from build123d import *

# Parameters (mm, degrees)
F0_R     = 33.4136580184
F1_DEPTH = 38.0875840783
F3_R     = 0.3813665803


with BuildPart() as f1:
    # F0 (on Top) → F1 (new body)
    with BuildSketch(Plane.XY):
        Circle(F0_R)
    extrude(amount=F1_DEPTH)

    # F2: F1 across plane


with BuildPart() as f1_1:
    add(f1.part)
    add(f1.part.mirror(Plane.XY))

    # F3
    f3_edges = [f1_1.edges().sort_by_distance(p)[0] for p in [
        (-33.413658, 0, -38.087584),
        (-33.413658, 0, 38.087584),
    ]]
    fillet(f3_edges, radius=F3_R)


solid = f1_1.part
Can you work these out from the model? Positions are in its coordinate system, mm. Give positions to 0.01 mm unless a question says otherwise; leave off trailing zeros. Loops run counter-clockwise (first coordinate to the right, second up) from the corner with the lowest first, then second, coordinate; pieces in that order, holes last. Notation, with made-up numbers: (-40, 67.25) -> (-35, 67.25) arc R8 cw to (-35, 79.25) -> close; hole circle Ø3 at (32, 49.25). An arc over 180 degrees is marked (long way). Write item = value, one per line.
1) Will these pins go through, and if not, where does the flat tip stop? pin 1 (10 mm diameter, centred on x = -13.5, z = -20.5, fed in from +Y); pin 2 (8 mm diameter, centred on y = 17, z = -23, fed in from +X); pin 3 (12 mm diameter, centred on y = 12.5, z = -22.5, fed in from +X).
Check result:
pin_1 = 32.31
pin_2 = 30.78
pin_3 = 32.78
2) I need wall thicknesses on L1, parallel to Y at x = -5, z = -14.5; L2, parallel to Y at x = 2, z = 3. Which ranges of each line are inside material? Lowest first, please. Write a range as from..to.
Check result:
L1 = -33.04..33.04
L2 = -33.35..33.35
3) Suppose I cut it at A-A on z = -13. Write out the boundary of the cut face in (x, y).
Check result:
outline = circle Ø66.83 at (0, 0)
4) Thinking about a two-plate mould opening in Y: for faces 1 (the flat face through (0, 0, -38.088)), 2 (the cylindrical face through (-26.516, -20.332, 0.528)), which applies, released by +Y, released by -Y, zero draft, split by the parting line, or undercut?
Check result:
face_1 = zero draft
face_2 = split by the parting line
